For this review, take the finished solid that the model builds, in its own axes (mm). Coordinates: 2 decimals unless noted, no trailing zeros. Write each loop counter-clockwise with the first axis right and the second up, starting at its lowest first coordinate (ties: lowest second). Pieces come first, ordered by that corner, then holes.
```python
from build123d import *

# Parameters (mm, degrees)
SKETCH_W            = 22.5
SKETCH_H            = 18
PAD_DEPTH           = 0.8
SKETCH001_R         = 1.1
POCKET_DEPTH        = 5
FILLET_R            = 1
SKETCH002_R         = 0.6
POCKET001_DEPTH     = 5
LINEARPATTERN_COUNT = 4
LINEARPATTERN_PITCH = 3.666667


with BuildPart() as part:
    # Sketch → Pad (new body)
    with BuildSketch(Plane.XZ):
        with Locations((11.25, 9)):
            Rectangle(SKETCH_W, SKETCH_H)
    extrude(amount=PAD_DEPTH)

    # Sketch001 (on Face6 of Pad) → Pocket (cut)
    with BuildSketch(Plane.XZ.offset(0.8)):
        with Locations((3, 15)):
            Circle(SKETCH001_R)
        with Locations((3, 3)):
            Circle(SKETCH001_R)
    extrude(amount=-POCKET_DEPTH, mode=Mode.SUBTRACT)

    # Fillet
    fillet_edges = [part.edges().sort_by_distance(p)[0] for p in [
        (0, -0.4, 18),
        (22.5, -0.4, 18),
        (22.5, -0.4, 0),
        (0, -0.4, 0),
    ]]
    fillet(fillet_edges, radius=FILLET_R)

    # Sketch002 (on Face5 of Fillet) → Pocket001 (cut)
    with BuildSketch(Plane.XZ.offset(0.8)):
        with Locations((7.5, 15)):
            Circle(SKETCH002_R)
        with Locations((7.5, 3)):
            Circle(SKETCH002_R)
    pocket001 = extrude(amount=-POCKET001_DEPTH, mode=Mode.SUBTRACT)

    # LinearPattern: Pocket001 ×4
    with Locations(*[(i * LINEARPATTERN_PITCH, 0, 0) for i in range(1, LINEARPATTERN_COUNT)]):
        add(pocket001, mode=Mode.SUBTRACT)


solid = part.part
```
Q1. Draft analysis for pull direction Z (two halves, no side actions). For faces 1 (the cylindrical face through (0.285, -0.406, 17.699)), 2 (the cylindrical face through (0.285, -0.406, 0.301)), 3 (the cylindrical face through (15.4, -0.4, 2.8)), 4 (the cylindrical face through (10.724, -0.406, 15.406)), state which applies: +Z half, -Z half, draft (parallel to the pull), parting line (faces both ways), or undercut.
Ans:
face 1: +Z half
face 2: -Z half
face 3: undercut
face 4: undercut
Q2. Add section B-B (y = -0.25). Give the number of separate pieces and of enclosed holes in the cut face, then the cut area to 3 significant figures.
Ans:
separate pieces: 1
enclosed holes: 10
area: 387 mm2
Q3. Add section D-D (x = 3). State the section outline as (y, z) points.
Ans:
outline: (-0.8, 0) - (0, 0) - (0, 1.9) - (-0.8, 1.9) - close; (-0.8, 4.1) - (0, 4.1) - (0, 13.9) - (-0.8, 13.9) - close; (-0.8, 16.1) - (0, 16.1) - (0, 18) - (-0.8, 18) - close
Q4. Add section A-A (x = 7.5). State the section outline as (y, z) points, then the cut area to 3 significant figures.
Ans:
outline: (-0.8, 0) - (0, 0) - (0, 2.4) - (-0.8, 2.4) - close; (-0.8, 3.6) - (0, 3.6) - (0, 14.4) - (-0.8, 14.4) - close; (-0.8, 15.6) - (0, 15.6) - (0, 18) - (-0.8, 18) - close
area: 12.5 mm2
Q5. For probe 1 along Z at (x, y) = (3, -0.4); probe 2 along Z at (x, y) = (7.5, -0.15); probe 3 along X at (y, z) = (-0.1, 14.75), list the stretches that pass through material, from the lowest coordinate up.
Ans:
probe 1: z = 0 to 1.9, 4.1 to 13.9, 16.1 to 18
probe 2: z = 0 to 2.4, 3.6 to 14.4, 15.6 to 18
probe 3: x = 0 to 1.93, 4.07 to 6.95, 8.05 to 10.62, 11.71 to 14.29, 15.38 to 17.95, 19.05 to 22.5
Q6. Clearance check with a flat-ended pin moving along its axis: pin 1 Ø0.7 at (x, z) = (11.17, 15) entering from +Y. State where the tip first meets the part, or that it passes through.
Ans:
pin 1: passes through
Q7. Add section C-C (z = 15). State the section outline as (x, y) points, then the cut area to 3 significant figures.
Ans:
outline: (0, -0.8) - (1.9, -0.8) - (1.9, 0) - (0, 0) - close; (4.1, -0.8) - (6.9, -0.8) - (6.9, 0) - (4.1, 0) - close; (8.1, -0.8) - (10.57, -0.8) - (10.57, 0) - (8.1, 0) - close; (11.77, -0.8) - (14.23, -0.8) - (14.23, 0) - (11.77, 0) - close; (15.43, -0.8) - (17.9, -0.8) - (17.9, 0) - (15.43, 0) - close; (19.1, -0.8) - (22.5, -0.8) - (22.5, 0) - (19.1, 0) - close
area: 12.4 mm2
